Source: CAD feature listing. Evaluate the final solid. Frame: model axes, mm. Face numbers are marked on the shaded views. A direction names the side the tool comes from. Round coordinates to 2 decimals unless told otherwise and drop trailing zeros. Loops run counter-clockwise (first coordinate to the right, second up) from the corner with the lowest first, then second, coordinate; pieces in that order, holes last. Notation, with made-up numbers: (79, -10.75) -> (133, -10.75) arc R10 cw to (133, 3.25) -> close; hole circle Ø7 at (57, 76.5). An arc over 180 degrees is marked (long way). Return JSON: item names as keys, results as strings. Group by question number.
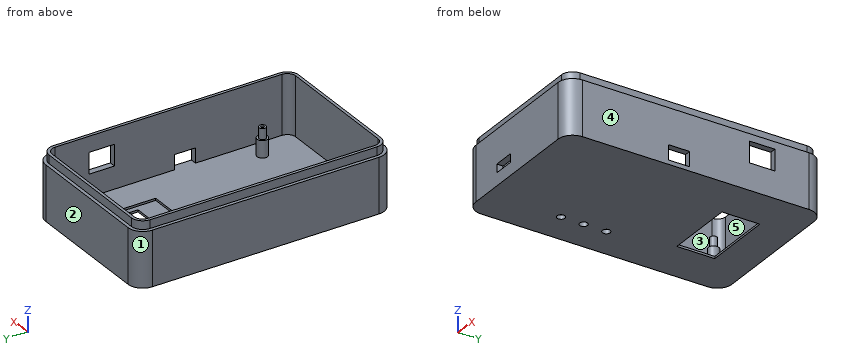
```python
from build123d import *

# Parameters (mm, degrees)
PAD_DEPTH         = 2
SKETCH004_W       = 38
SKETCH004_H       = 35
POCKET_DEPTH      = 1
SKETCH003_W       = 33
SKETCH003_H       = 18
POCKET001_DEPTH   = 2
SKETCH005_R       = 1.85
POCKET002_DEPTH   = 2
SKETCH006_R       = 2.5
PAD001_DEPTH      = 10
SKETCH007_R       = 1.65
PAD002_DEPTH      = 15
PAD003_DEPTH      = 26
PAD004_DEPTH      = 30
CYLINDER_R        = 0.75
CYLINDER_DEPTH    = 10
CYLINDER001_R     = 0.75
CYLINDER001_DEPTH = 10
CYLINDER002_R     = 0.75
CYLINDER002_DEPTH = 10
CYLINDER003_R     = 0.75
CYLINDER003_DEPTH = 10
SKETCH008_W       = 3
SKETCH008_H       = 12
POCKET003_DEPTH   = 10
BOX_W             = 4
BOX_H             = 10
BOX_DEPTH         = 7
SKETCH009_W       = 10.000002
SKETCH009_H       = 3
POCKET004_DEPTH   = 4


with BuildPart() as part:
    # Sketch → Pad (new body)
    with BuildSketch(Plane.XY):
        with BuildLine():
            Line((0, 114.650046), (0, 7))
            ThreePointArc((0, 7), (2.050253, 2.050253), (7, 0))
            Line((7, 0), (67.149994, 0))
            ThreePointArc((67.149994, 0), (72.099741, 2.050253), (74.149994, 7))
            Line((74.149994, 7), (74.149994, 114.650046))
            ThreePointArc((74.149994, 114.650046), (72.099741, 119.599793), (67.149994, 121.650046))
            Line((67.149994, 121.650046), (7, 121.650046))
            ThreePointArc((7, 121.650046), (2.050253, 119.599793), (0, 114.650046))
        make_face()
    extrude(amount=PAD_DEPTH)

    # Sketch004 → Pocket (cut)
    with BuildSketch(Plane.XY.offset(2)):
        with Locations((37.074997, 94.150046)):
            Rectangle(SKETCH004_W, SKETCH004_H)
    extrude(amount=-POCKET_DEPTH, mode=Mode.SUBTRACT)

    # Sketch003 → Pocket001 (cut)
    with BuildSketch(Plane.XY.offset(2)):
        with Locations((37.074997, 95.650046)):
            Rectangle(SKETCH003_W, SKETCH003_H)
    extrude(amount=-POCKET001_DEPTH, mode=Mode.SUBTRACT)

    # Sketch005 → Pocket002 (cut)
    with BuildSketch(Plane.XY.offset(2)):
        with Locations((15.325171, 35.075006)):
            Circle(SKETCH005_R)
        with Locations((15.325058, 45.825065)):
            Circle(SKETCH005_R)
        with Locations((15.325117, 56.575053)):
            Circle(SKETCH005_R)
    extrude(amount=-POCKET002_DEPTH, mode=Mode.SUBTRACT)

    # Sketch006 → Pad001 (join)
    with BuildSketch(Plane.XY):
        with Locations((62.075039, 22.075116)):
            Circle(SKETCH006_R)
        with Locations((12.075062, 22.075062)):
            Circle(SKETCH006_R)
        with Locations((12.075024, 109.57503)):
            Circle(SKETCH006_R)
        with Locations((62.075044, 109.575056)):
            Circle(SKETCH006_R)
    extrude(amount=PAD001_DEPTH)

    # Sketch007 → Pad002 (join)
    with BuildSketch(Plane.XY):
        with Locations((62.075039, 22.075116)):
            Circle(SKETCH007_R)
        with Locations((12.075062, 22.075062)):
            Circle(SKETCH007_R)
        with Locations((62.075044, 109.575056)):
            Circle(SKETCH007_R)
        with Locations((12.075024, 109.57503)):
            Circle(SKETCH007_R)
    extrude(amount=PAD002_DEPTH)

    # Sketch001 → Pad003 (join)
    with BuildSketch(Plane.XY):
        with BuildLine():
            Line((0, 114.650046), (0, 7))
            ThreePointArc((0, 7), (2.050253, 2.050253), (7, 0))
            Line((7, 0), (67.149994, 0))
            ThreePointArc((67.149994, 0), (72.099741, 2.050253), (74.149994, 7))
            Line((74.149994, 7), (74.149994, 114.650046))
            ThreePointArc((74.149994, 114.650046), (72.099741, 119.599793), (67.149994, 121.650046))
            Line((67.149994, 121.650046), (7, 121.650046))
            ThreePointArc((7, 121.650046), (2.050253, 119.599793), (0, 114.650046))
        make_face()
        with BuildLine():
            Line((67.149994, 118.650046), (7, 118.650046))
            ThreePointArc((7, 118.650046), (4.171573, 117.478473), (3, 114.650046))
            Line((3, 114.650046), (3, 7))
            ThreePointArc((3, 7), (4.171573, 4.171573), (7, 3))
            Line((7, 3), (67.149994, 3))
            ThreePointArc((67.149994, 3), (69.978421, 4.171573), (71.149994, 7))
            Line((71.149994, 7), (71.149994, 114.650046))
            ThreePointArc((71.149994, 114.650046), (69.978421, 117.478473), (67.149994, 118.650046))
        make_face(mode=Mode.SUBTRACT)
    extrude(amount=PAD003_DEPTH)

    # Sketch002 → Pad004 (join)
    with BuildSketch(Plane.XY):
        with BuildLine():
            Line((67.149994, 120.050046), (7, 120.050046))
            ThreePointArc((7, 120.050046), (3.181623, 118.468423), (1.6, 114.650046))
            Line((1.6, 114.650046), (1.6, 7))
            ThreePointArc((1.6, 7), (3.181623, 3.181623), (7, 1.6))
            Line((7, 1.6), (67.149994, 1.6))
            ThreePointArc((67.149994, 1.6), (70.968371, 3.181623), (72.549994, 7))
            Line((72.549994, 7), (72.549994, 114.650046))
            ThreePointArc((72.549994, 114.650046), (70.968371, 118.468423), (67.149994, 120.050046))
        make_face()
        with BuildLine():
            Line((67.149994, 118.650046), (7, 118.650046))
            ThreePointArc((7, 118.650046), (4.171573, 117.478473), (3, 114.650046))
            Line((3, 114.650046), (3, 7))
            ThreePointArc((3, 7), (4.171573, 4.171573), (7, 3))
            Line((7, 3), (67.149994, 3))
            ThreePointArc((67.149994, 3), (69.978421, 4.171573), (71.149994, 7))
            Line((71.149994, 7), (71.149994, 114.650046))
            ThreePointArc((71.149994, 114.650046), (69.978421, 117.478473), (67.149994, 118.650046))
        make_face(mode=Mode.SUBTRACT)
    extrude(amount=PAD004_DEPTH)

    # Cylinder → Cylinder (cut)
    with BuildSketch(Plane(origin=(12.075062, 22.075062, 15), x_dir=(-1, 0, 0), z_dir=(0, 0, -1))):
        Circle(CYLINDER_R)
    extrude(amount=CYLINDER_DEPTH, mode=Mode.SUBTRACT)

    # Cylinder001 → Cylinder001 (cut)
    with BuildSketch(Plane(origin=(62.075039, 22.075116, 15), x_dir=(-1, 0, 0), z_dir=(0, 0, -1))):
        Circle(CYLINDER001_R)
    extrude(amount=CYLINDER001_DEPTH, mode=Mode.SUBTRACT)

    # Cylinder002 → Cylinder002 (cut)
    with BuildSketch(Plane(origin=(62.075044, 109.575056, 15), x_dir=(-1, 0, 0), z_dir=(0, 0, -1))):
        Circle(CYLINDER002_R)
    extrude(amount=CYLINDER002_DEPTH, mode=Mode.SUBTRACT)

    # Cylinder003 → Cylinder003 (cut)
    with BuildSketch(Plane(origin=(12.075024, 109.57503, 15), x_dir=(-1, 0, 0), z_dir=(0, 0, -1))):
        Circle(CYLINDER003_R)
    extrude(amount=CYLINDER003_DEPTH, mode=Mode.SUBTRACT)

    # Sketch008 → Pocket003 (cut)
    with BuildSketch(Plane.XY.offset(12.6)):
        with Locations((72.649994, 92.446222)):
            Rectangle(SKETCH008_W, SKETCH008_H)
    extrude(amount=POCKET003_DEPTH, mode=Mode.SUBTRACT)

    # Box → Box (cut)
    with BuildSketch(Plane(origin=(70.192996, 47.991786, 2), x_dir=(0.999999, 0.001479, 0), z_dir=(0, 0, 1))):
        with Locations((2, 5)):
            Rectangle(BOX_W, BOX_H)
    extrude(amount=BOX_DEPTH, mode=Mode.SUBTRACT)

    # Sketch009 → Pocket004 (cut)
    with BuildSketch(Plane.XY.offset(6)):
        with Locations((27.364886, 1.5)):
            Rectangle(SKETCH009_W, SKETCH009_H)
    extrude(amount=POCKET004_DEPTH, mode=Mode.SUBTRACT)


solid = part.part
```
(1) Pin query (flat end, axial travel): pin 1 (1.2 mm diameter, centred on x = 12.5, y = 22.5, fed in from +Z); pin 2 (3.5 mm diameter, centred on y = 2, z = 8, fed in from -X); pin 3 (1.4 mm diameter, centred on x = 12.08, y = 22.08, fed in from +Z). Return the tip coordinate at first contact, or that it passes through.
(2) Cut plane B-B (x = 35.5). Return loops of the section in (y, z).
(3) Cut plane D-D (y = 51.5). Return loops of the section in (x, z).
(4) Cut plane A-A (y = 88). Return loops of the section in (x, z) (3 decimals).
(5) Mould query, pull axis X, two halves, no side actions, for the marked faces 1, 2 and 3. Classes: released by +X, released by -X, zero draft, split by the parting line, or undercut.
(6) Ray query, line 1 (Y direction, x = 47.5, z = 5); line 2 (X direction, y = 14, z = 16); line 3 (X direction, y = 45, z = 27.25). Return the intervals inside material, ascending.
(7) Set-up query: the marked faces 4 and 5. Return all of +Z, -Z, +X, -X, +Y, -Y with unobstructed straight access to the full face (end or side cutting, diameter ignored); none if empty.
(8) Cut plane C-C (z = 7.25). Count the separate pieces of the cut face and the enclosed holes in it, and give its area (3 significant figures).
Answers follow:
{
 "1": {"pin 1": "z = 15", "pin 2": "x = 0.8", "pin 3": "z = 5"},
 "2": {"outline": "(0, 0) -> (86.65, 0) -> (86.65, 1) -> (76.65, 1) -> (76.65, 2) -> (3, 2) -> (3, 30) -> (1.6, 30) -> (1.6, 26) -> (0, 26) -> close; (104.65, 0) -> (121.65, 0) -> (121.65, 26) -> (120.05, 26) -> (120.05, 30) -> (118.65, 30) -> (118.65, 2) -> (111.65, 2) -> (111.65, 1) -> (104.65, 1) -> close"},
 "3": {"outline": "(0, 0) -> (74.15, 0) -> (74.15, 2) -> (3, 2) -> (3, 30) -> (1.6, 30) -> (1.6, 26) -> (0, 26) -> close; (71.15, 9) -> (74.15, 9) -> (74.15, 26) -> (72.55, 26) -> (72.55, 30) -> (71.15, 30) -> close"},
 "4": {"outline": "(0, 0) -> (20.575, 0) -> (20.575, 1) -> (18.075, 1) -> (18.075, 2) -> (3, 2) -> (3, 30) -> (1.6, 30) -> (1.6, 26) -> (0, 26) -> close; (53.575, 0) -> (74.15, 0) -> (74.15, 12.6) -> (71.15, 12.6) -> (71.15, 2) -> (56.075, 2) -> (56.075, 1) -> (53.575, 1) -> close; (71.15, 22.6) -> (74.15, 22.6) -> (74.15, 26) -> (72.55, 26) -> (72.55, 30) -> (71.15, 30) -> close"},
 "5": {"face 1": "released by -X", "face 2": "zero draft", "face 3": "undercut"},
 "6": {"line 1": "0 to 3, 118.65 to 121.65", "line 2": "0 to 3, 71.15 to 74.15", "line 3": "1.6 to 3, 71.15 to 72.55"},
 "7": {"face 4": "+Z, -Z, +X, +Y, -Y", "face 5": "+Z"},
 "8": {"separate pieces": "6", "enclosed holes": "4", "area": "1,120 mm^2"}
}
